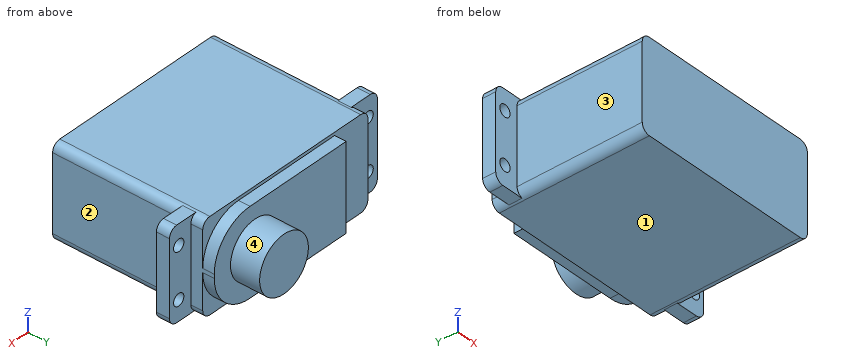
```python
from build123d import *

# Parameters (mm, degrees)
SKETCH1_W           = 58.674
SKETCH1_H           = 28.5242
BOSS_EXTRUDE1_DEPTH = 46.609
SKETCH2_W           = 46.863
SKETCH2_H           = 26.6192
BOSS_EXTRUDE2_DEPTH = 3.5814
FILLET1_R           = 12.7
FILLET2_R           = 2.54
BOSS_EXTRUDE3_START = -7.747
SKETCH3_W           = 73.8632
SKETCH3_H           = 28.2702
BOSS_EXTRUDE3_DEPTH = 4.064
FILLET3_R           = 2.54
SKETCH4_R           = 1.8288
CUT_EXTRUDE1_DEPTH  = 43.926
SKETCH5_R           = 8.6614
BOSS_EXTRUDE4_DEPTH = 12.6238


with BuildPart() as part:
    # Sketch1 → Boss-Extrude1 (new body)
    with BuildSketch(Plane(origin=(0, 0, 0), x_dir=(1, 0, 0), z_dir=(0, 1, 0))):
        Rectangle(SKETCH1_W, SKETCH1_H)
    extrude(amount=BOSS_EXTRUDE1_DEPTH)

    # Sketch2 → Boss-Extrude2 (add)
    with BuildSketch(Plane(origin=(0, 46.609, 0), x_dir=(1, 0, 0), z_dir=(0, 1, 0))):
        with Locations((5.9055, 0)):
            Rectangle(SKETCH2_W, SKETCH2_H)
    extrude(amount=BOSS_EXTRUDE2_DEPTH)

    # Fillet1
    fillet1_edges = [part.edges().sort_by_distance(p)[0] for p in [
        (29.337, 48.3997, 13.3096),
        (29.337, 48.3997, -13.3096),
    ]]
    fillet(fillet1_edges, radius=FILLET1_R)

    # Fillet2
    fillet2_edges = [part.edges().sort_by_distance(p)[0] for p in [
        (29.337, 23.3045, 14.2621),
        (29.337, 23.3045, -14.2621),
        (-29.337, 23.3045, -14.2621),
        (-29.337, 23.3045, 14.2621),
    ]]
    fillet(fillet2_edges, radius=FILLET2_R)

    # Sketch3 → Boss-Extrude3 (add)
    with BuildSketch(Plane(origin=(0, 46.609, 0), x_dir=(1, 0, 0), z_dir=(0, 1, 0)).offset(BOSS_EXTRUDE3_START)):
        Rectangle(SKETCH3_W, SKETCH3_H)
    extrude(amount=BOSS_EXTRUDE3_DEPTH)

    # Fillet3
    fillet3_edges = [part.edges().sort_by_distance(p)[0] for p in [
        (36.9316, 40.894, -14.1351),
        (-36.9316, 40.894, -14.1351),
        (-36.9316, 40.894, 14.1351),
        (36.9316, 40.894, 14.1351),
    ]]
    fillet(fillet3_edges, radius=FILLET3_R)

    # Sketch4 → Cut-Extrude1 (cut, through all)
    with BuildSketch(Plane(origin=(0, 42.926, 0), x_dir=(1, 0, 0), z_dir=(0, 1, 0))):
        with Locations((-33.655, 7.874)):
            Circle(SKETCH4_R)
        with Locations((-33.655, -7.874)):
            Circle(SKETCH4_R)
        with Locations((33.655, -7.874)):
            Circle(SKETCH4_R)
        with Locations((33.655, 7.874)):
            Circle(SKETCH4_R)
    extrude(amount=-CUT_EXTRUDE1_DEPTH, mode=Mode.SUBTRACT)

    # Sketch5 → Boss-Extrude4 (add)
    with BuildSketch(Plane(origin=(0, 46.609, 0), x_dir=(1, 0, 0), z_dir=(0, 1, 0))):
        with Locations((14.9098, 0)):
            Circle(SKETCH5_R)
    extrude(amount=BOSS_EXTRUDE4_DEPTH)


solid = part.part
```
Source: CAD feature listing. Evaluate the final solid. Frame: model axes, mm. Face numbers are marked on the shaded views. A direction names the side the tool comes from. Give positions to 0.01 mm unless a question says otherwise; leave off trailing zeros. Loops run counter-clockwise (first coordinate to the right, second up) from the corner with the lowest first, then second, coordinate; pieces in that order, holes last. Notation, with made-up numbers: (-1, 17.25) - (25, 17.25) arc R11 ccw to (25, 31.25) - close; hole circle Ø9 at (26.25, 11.25). An arc over 180 degrees is marked (long way). Use CSV: the item, a comma, the result in double quotes. Start each with the question number.
1. Pin query (flat end, axial travel): pin 1 (10.5 mm diameter, centred on x = -33, z = -2.5, fed in from +Y); pin 2 (3 mm diameter, centred on x = -33.655, z = -7.874, fed in from +Y); pin 3 (6 mm diameter, centred on x = -33.655, z = 7.874, fed in from +Y); pin 4 (1.8 mm diameter, centred on y = 44.5, z = -1.5, fed in from -X). Return the tip coordinate at first contact, or that it passes through.
2. Reachability of the marked faces 1, 2, 3 and 4 from +Z, -Z, +X, -X, +Y, -Y: full face, straight path, thin tool, end or side. Return the list, or none.
3. Section B-B (x = -3). Output: boundary loops of the cut face in (y, z).
4. Section C-C (z = -3.75). Output: boundary loops of the cut face in (x, y).
5. Section A-A (y = 22.5). Output: boundary loops of the cut face in (x, z).
6. Section D-D (x = 14.5). Output: boundary loops of the cut face in (y, z).
7. Ray query, L1, parallel to X at y = 20, z = -7.25; L2, parallel to Y at x = -22, z = 5; L3, parallel to X at y = 42.5, z = 7. Return the intervals inside material, ascending.
Response:
1,pin 1,"y = 46.61"
1,pin 2,"through"
1,pin 3,"y = 42.93"
1,pin 4,"x = -29.34"
2,face 1,"-Z, +X, -X, +Y, -Y"
2,face 2,"+Z, -Z, +X, -Y"
2,face 3,"+Z, -Z, -X, -Y"
2,face 4,"+Y"
3,outline,"(0, -14.26) - (46.61, -14.26) - (46.61, -13.31) - (50.19, -13.31) - (50.19, 13.31) - (46.61, 13.31) - (46.61, 14.26) - (0, 14.26) - close"
4,outline,"(-36.93, 38.86) - (-29.34, 38.86) - (-29.34, 0) - (29.34, 0) - (29.34, 38.86) - (36.93, 38.86) - (36.93, 42.93) - (29.34, 42.93) - (29.34, 46.61) - (28.94, 46.61) - (28.94, 50.19) - (22.72, 50.19) - (22.72, 59.23) - (7.1, 59.23) - (7.1, 50.19) - (-17.53, 50.19) - (-17.53, 46.61) - (-29.34, 46.61) - (-29.34, 42.93) - (-36.93, 42.93) - close"
5,outline,"(-29.34, -11.72) arc R2.54 ccw to (-26.8, -14.26) - (26.8, -14.26) arc R2.54 ccw to (29.34, -11.72) - (29.34, 11.72) arc R2.54 ccw to (26.8, 14.26) - (-26.8, 14.26) arc R2.54 ccw to (-29.34, 11.72) - close"
6,outline,"(0, -14.26) - (46.61, -14.26) - (46.61, -13.31) - (50.19, -13.31) - (50.19, -8.65) - (59.23, -8.65) - (59.23, 8.65) - (50.19, 8.65) - (50.19, 13.31) - (46.61, 13.31) - (46.61, 14.26) - (0, 14.26) - close"
7,L1,"-29.34 to 29.34"
7,L2,"0 to 46.61"
7,L3,"-36.93 to -35.26, -32.05 to 32.05, 35.26 to 36.93"
